Check sheet for the modelled part. Datum: model origin and axes. Units: mm. Face numbers are marked on the shaded views. Round coordinates to 2 decimals unless told otherwise and drop trailing zeros. Order: outer loops, then holes, each group sorted by start corner. A loop starts at its lowest first (then second) coordinate and runs counter-clockwise, first axis right, second up. Notation, with made-up numbers: (80, 89.5) -> (136, 89.5) arc R30 cw to (136, 128.5) -> close; hole circle Ø10 at (58, 14.5). An arc over 180 degrees is marked (long way). Answer in a Markdown table with one row per item.
Autodesk Inventor part; units mm, degrees
ref_plane "YZ Plane" through (0, 0, 0) normal (1, 0, 0) x (0, 1, 0)
ref_plane "XZ Plane" through (0, 0, 0) normal (0, 1, 0) x (-1, 0, 0)
ref_plane "XY Plane" through (0, 0, 0) normal (0, 0, 1) x (1, 0, 0)
sketch "Эскиз1" plane through (0, 0, 0) normal (0, 0, 1) x (1, 0, 0)
  circle A0 centre (0, 0) radius 40
  circle A1 centre (0, 0) radius 22.5
  dimension "d0" = 80
  dimension "d1" = 45
extrude "Выдавливание1" add sketch "Эскиз1" along normal blind 30
sketch "Эскиз2" plane through (0, 0, 0) normal (1, 0, 0) x (0, 1, 0)
  line L0 (40, 0) -> (-40, 0)
  line L1 (22.5, 30) -> (22.5, 0)
  line L2 (22.5, 0) -> (22.5, -6)
  line L3 (22.5, -6) -> (27.5, -6)
  arc A0 (32.491841, 1.501959) -> (29.238817, 0.515685) centre (31.17119, 0) ccw
  line L4 (27.5, -6) -> (29.238817, 0.515685)
  line L5 (34.2, 0) -> (32.491841, 1.501959)
  line L6 (0, -13.2) -> (0, 37.2)
  point P0 (0, 0)
  point P1 (29.101198, 0)
  dimension "d4" = 5
  dimension "d5" = 6
  dimension "d6" = 4
  dimension "d9" = 27.5
  dimension "d10" = 29.23882
revolve "Вращение1" add sketch "Эскиз2" angle 360 about axis through (0, 0, -10) along (0, 0, 1) contours L4 L3 L2 L0
revolve "Вращение2" cut sketch "Эскиз2" angle 360 about axis through (0, 0, -10) along (0, 0, 1) contours L0 L4 A0 L5
chamfer "Фаска1" distance 2 angle 45 2 edges at (0, -22.5, -6) (-22.5, 0, 30)
sketch "Эскиз3" plane through (0, 0, 0) normal (1, 0, 0) x (0, 1, 0)
  line L0 (40, 0) -> (40, 30)
  line L1 (40, 15) -> (26.875653, 15)
  line L2 (40, 15) -> (40, 20)
  line L3 (40, 20) -> (30, 20)
  line L4 (30, 20) -> (26.606861, 14.569843)
  point P0 (0, 0)
  dimension "d14" = 10
  dimension "d15" = 58
revolve "Вращение3" cut sketch "Эскиз3" angle 360 about axis through (0, 40, 15) along (0, -1, 0)
thread "Резьба1"
properties part number "Гайка шток_CPY" material "Сталь, высокопрочная, низколегированная"
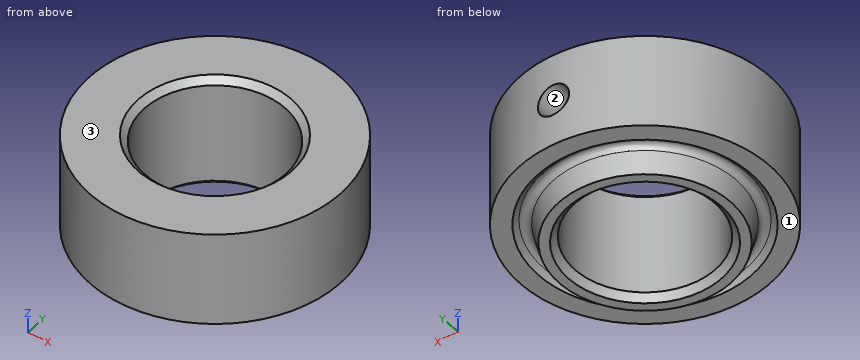
Item 1: Mould release check, pull along Z, two halves, no side actions. Record for the marked faces 1, 2 and 3: pulls with the +Z half, pulls with the -Z half, needs draft (parallel to the pull), parting line crosses it, or undercut.
Result sheet:
| item | result |
|---|---|
| face 1 | pulls with the -Z half |
| face 2 | undercut |
| face 3 | pulls with the +Z half |
Item 2: Cross-section at A-A (z = 7). Record the boundary of the cut face in (x, y).
Result sheet:
| item | result |
|---|---|
| outline | circle Ø80 at (0, 0); hole circle Ø45 at (0, 0) |
Item 3: Depth check by flat-ended pin: P1, Ø5, axis at y = -13.5, z = 26, coming from the -X side; P2, Ø8, axis at x = 0, z = 15, coming from the +Y side; P3, Ø8, axis at y = 8.5, z = 11, coming from the -X side. Enter the tip coordinate at first touch or a pass-through.
Result sheet:
| item | result |
|---|---|
| P1 | stops at x = -38.46 |
| P2 | stops at y = 29.38 |
| P3 | stops at x = -39.75 |
Item 4: Scan lines: line 1 (Y direction, x = 0, z = 9); line 2 (Y direction, x = 0, z = 16); line 3 (X direction, y = -20, z = 12). Record each from-to range of solid material in increasing order. Write a range as [from, to].
Result sheet:
| item | result |
|---|---|
| line 1 | y = [-40, -22.5], [22.5, 40] |
| line 2 | y = [-40, -22.5], [22.5, 27.5] |
| line 3 | x = [-34.64, -10.31], [10.31, 34.64] |
